```python
from build123d import *

# Parameters (mm, degrees)
F0_W     = 58
F0_H     = 127
F1_DEPTH = 3.175
F2_W     = 3.075
F2_H     = 21.2
F2_W_2   = 9.9
F2_H_2   = 3.075
F3_DEPTH = 25


# Not quite as in the source:
# - a length typed as a fraction of an inch, garbled in the dataset ("3 / 203.2 mm" for 3/8 in), is restored


with BuildPart() as f1:
    # F0 (on Front) → F1 (new body)
    with BuildSketch(Plane.XZ):
        Rectangle(F0_W, F0_H)
    extrude(amount=F1_DEPTH)

    # F2 (on face) → F3 (cut)
    with BuildSketch(Plane(origin=(0, 0, 0), x_dir=(-1, 0, 0), z_dir=(0, 1, 0))):
        Polygon((-19.1, 63.5), (-29, 63.5), (-29, 53.6), (-25.925, 53.6), (-25.925, 60.425), (-19.1, 60.425), align=None)
        with Locations((-27.4625, 21.4)):
            Rectangle(F2_W, F2_H)
        with Locations((-27.4625, -21.4)):
            Rectangle(F2_W, F2_H)
        Polygon((-25.925, -53.6), (-29, -53.6), (-29, -63.5), (-19.1, -63.5), (-19.1, -60.425), (-25.925, -60.425), align=None)
        with Locations((24.05, 61.9625)):
            Rectangle(F2_W_2, F2_H_2)
        with Locations((24.05, -61.9625)):
            Rectangle(F2_W_2, F2_H_2)
    extrude(amount=-F3_DEPTH, mode=Mode.SUBTRACT)


solid = f1.part
```
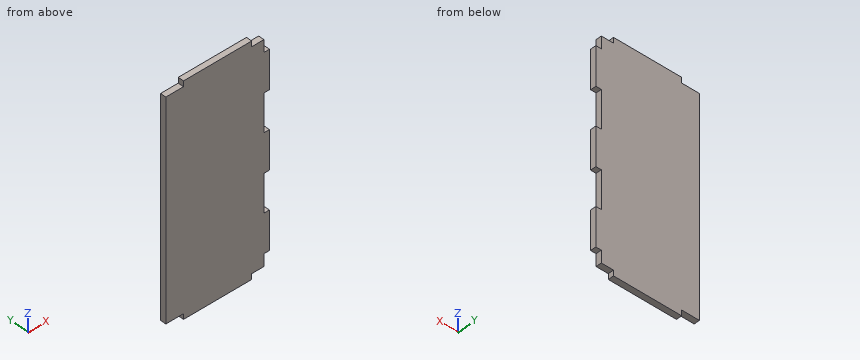
Could you check a few things on this model? Use its own coordinates, in mm. Round coordinates to 2 decimals unless told otherwise and drop trailing zeros. Write each loop counter-clockwise with the first axis right and the second up, starting at its lowest first coordinate (ties: lowest second). Pieces come first, ordered by that corner, then holes. Notation, with made-up numbers: M 23.25,-35 L 29.25,-35 A23 ccw 29.25,-12 Z; hole C 28.5,33 d8. An arc over 180 degrees is marked long. Answer in a Markdown table with one row per item. Add a question column.
Q1. Will these pins go through, and if not, where does the flat tip stop? pin 1 Ø1.5 at (x, y) = (27.5, -2) entering from -Z; pin 2 Ø0.9 at (y, z) = (-2, 62.5) entering from -X; pin 3 Ø1.5 at (x, z) = (4, -15) entering from +Y; pin 4 Ø1.6 at (x, y) = (-26.5, -1) entering from +Z (3 decimals).
Q2. If I drill on line 1 (Z direction, x = 26.5, y = -0.55); line 2 (X direction, y = -2.1, z = -13.5) (3 decimals); line 3 (Z direction, x = -19.5, y = -1.2) (3 decimals), over which ranges is the centre line in solid material (lowest first)? Write a range as from..to.
Q3. Imagine slicing it at A-A (y = -1). Please give me the cut outline in (x, z) (3 decimals), then the cut area to 3 significant figures.
Q4. Imagine slicing it at B-B (x = 20.5). Please give me the cut outline in (y, z) (3 decimals).
Values:
| question | item | result |
|---|---|---|
| 1 | pin 1 | z = -53.6 |
| 1 | pin 2 | x = -19.1 |
| 1 | pin 3 | y = 0 |
| 1 | pin 4 | z = 60.425 |
| 2 | line 1 | -53.6..-32, -10.8..10.8, 32..53.6 |
| 2 | line 2 | -29..25.925 |
| 2 | line 3 | -60.425..60.425 |
| 3 | outline | M -29,-60.425 L -19.1,-60.425 L -19.1,-63.5 L 19.1,-63.5 L 19.1,-60.425 L 25.925,-60.425 L 25.925,-53.6 L 29,-53.6 L 29,-32 L 25.925,-32 L 25.925,-10.8 L 29,-10.8 L 29,10.8 L 25.925,10.8 L 25.925,32 L 29,32 L 29,53.6 L 25.925,53.6 L 25.925,60.425 L 19.1,60.425 L 19.1,63.5 L -19.1,63.5 L -19.1,60.425 L -29,60.425 Z |
| 3 | area | 7,070 mm^2 |
| 4 | outline | M -3.175,-60.425 L 0,-60.425 L 0,60.425 L -3.175,60.425 Z |
